Answer from the drawing. Dimensions are ordinates in mm from the lowest x, y and z of the part. A direction names the side the tool comes from. Coordinates: 2 decimals unless noted, no trailing zeros. Order: outer loops, then holes, each group sorted by start corner. A loop starts at its lowest first (then second) coordinate and runs counter-clockwise, first axis right, second up. Notation, with made-up numbers: (-33, -37.5) - (-7, -37.5) arc R35 ccw to (-7, -0.5) - close; hole circle Ø3 at (21, 4). An arc over 180 degrees is marked (long way). One line per item, written item: value. Start each with the question number.
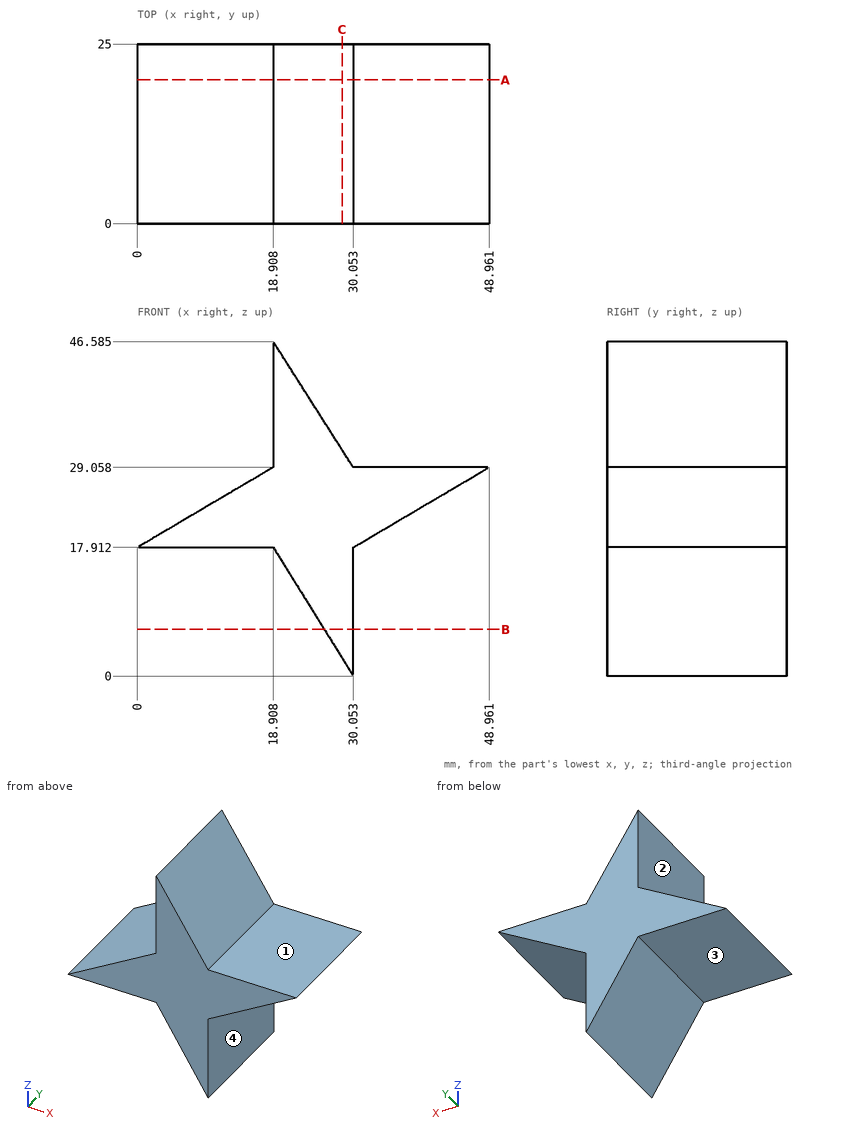
(1) The part is cut by section C-C on x = 28.5. Determine the outline of the cut face in (y, z), plus the area to 3 significant figures.
(2) For the marked faces 1, 2, 3 and 4, determine the directions among +Z, -Z, +X, -X, +Y, -Y from which every point of the face is accessible in a straight line to the end or side of a thin tool.
(3) Flat-ended cylindrical pins translate along their axes: pin 1 Ø1 at (y, z) = (15, 5) entering from +X; pin 2 Ø14 at (y, z) = (12.5, 40) entering from -X; pin 3 Ø10 at (y, z) = (18, 24) entering from +X (1 decimal); pin 4 Ø12 at (x, z) = (43.5, 40) entering from +Y. Find the tip coordinate at first contact, or state that the pin passes through.
(4) Consider probe 1 along Z at (x, y) = (12, 2) (1 decimal); probe 2 along X at (y, z) = (2.75, 42) (1 decimal); probe 3 along Z at (x, y) = (11, 8) (1 decimal). Determine where each line is inside the solid, lowest interval first.
(5) The part is cut by section B-B on z = 6.5. Determine the outline of the cut face in (x, y), plus the area to 3 significant figures.
(6) The part is cut by section A-A on y = 20. Determine the outline of the cut face in (x, z) (1 decimal).
Completed:
1. outline: (0, 2.5) - (25, 2.5) - (25, 31.5) - (0, 31.5) - close
1. area: 725 mm2
2. face 1: +Z, +X, +Y, -Y
2. face 2: +Z, -X, +Y, -Y
2. face 3: -Z, -X, +Y, -Y
2. face 4: -Z, +X, +Y, -Y
3. pin 1: stops at x = 30.05
3. pin 2: stops at x = 18.91
3. pin 3: stops at x = 48.9
3. pin 4: passes through
4. probe 1: z = 17.9 to 25
4. probe 2: x = 18.9 to 21.8
4. probe 3: z = 17.9 to 24.4
5. outline: (26.01, 0) - (30.05, 0) - (30.05, 25) - (26.01, 25) - close
5. area: 101 mm2
6. outline: (0, 17.9) - (18.9, 17.9) - (30.1, 0) - (30.1, 17.9) - (49, 29.1) - (30.1, 29.1) - (18.9, 46.6) - (18.9, 29.1) - close
